Source: CAD feature listing. Evaluate the final solid. Frame: model axes, mm. A direction names the side the tool comes from. Round coordinates to 2 decimals unless told otherwise and drop trailing zeros. Write each loop counter-clockwise with the first axis right and the second up, starting at its lowest first coordinate (ties: lowest second). Pieces come first, ordered by that corner, then holes. Notation, with made-up numbers: M 16,29 L 44,29 A28 ccw 44,65 Z; hole C -1.75,12 d7. An arc over 180 degrees is marked long. Use a Markdown table: item, result.
```python
from build123d import *

# Parameters (mm, degrees)
BOSS_EXTRUDE1_START = -2
SKETCH1_R           = 2.5
BOSS_EXTRUDE1_DEPTH = 5.5
BOSS_EXTRUDE2_REACH = 96.094
SKETCH2_R           = 5.5
SKETCH2_R_2         = 2.5
FILLET1_R           = 1.5


with BuildPart() as part:
    # Sketch1 → Boss-Extrude1 (new body)
    with BuildSketch(Plane(origin=(0, -76.733621845, 0), x_dir=(1, 0, 0), z_dir=(0, 1, 0)).offset(BOSS_EXTRUDE1_START)):
        with BuildLine():
            Line((52.941217068, 9.5), (69.945503657, 9.5))
            ThreePointArc((69.945503657, 9.5), (72.232982212, 8.946059138), (74.01360963, 7.406976744))
            Line((74.01360963, 7.406976744), (76.346988808, 4.141579527))
            ThreePointArc((76.346988808, 4.141579527), (82.014772389, 0.763045112), (88.341217068, 2.637708614))
            ThreePointArc((88.341217068, 2.637708614), (90.254455743, 4.667684765), (91.658842367, 7.07786808))
            Line((91.658842367, 7.07786808), (90.278524492, 7.07786808))
            ThreePointArc((90.278524492, 7.07786808), (89.953291089, 6.475468544), (89.591215146, 5.89446684))
            Line((89.591215146, 5.89446684), (88.341217068, 5.89446684))
            Line((88.341217068, 5.89446684), (88.341217068, 12))
            Line((88.341217068, 12), (88.341217068, 13.810660172))
            ThreePointArc((88.341217068, 13.810660172), (86.557690725, 18.116473657), (82.25187724, 19.9))
            Line((82.25187724, 19.9), (80.441217068, 19.9))
            ThreePointArc((80.441217068, 19.9), (76.827000951, 19.024773438), (74.01360963, 16.593023256))
            ThreePointArc((74.01360963, 16.593023256), (72.232982212, 15.053940862), (69.945503657, 14.5))
            Line((69.945503657, 14.5), (52.941217068, 14.5))
            ThreePointArc((52.941217068, 14.5), (50.441217068, 12), (52.941217068, 9.5))
        make_face()
        with Locations(Location((80.441217068, 12, 0), (0, 0, 270))):
            Circle(SKETCH1_R, mode=Mode.SUBTRACT)
    extrude(amount=-BOSS_EXTRUDE1_DEPTH)

    # Sketch2 → Boss-Extrude2 (add, up to next)
    with BuildSketch(Plane(origin=(0, -76.733621845, 0), x_dir=(-1, 0, 0), z_dir=(0, -1, 0)), mode=Mode.PRIVATE) as boss_extrude2_sk1:
        with Locations(Location((-80.441217068, 12, 0), (0, 0, 270))):
            Circle(SKETCH2_R)
        with Locations(Location((-80.441217068, 12, 0), (0, 0, 270))):
            Circle(SKETCH2_R_2, mode=Mode.SUBTRACT)
    boss_extrude2_tool1 = extrude(boss_extrude2_sk1.sketch, amount=BOSS_EXTRUDE2_REACH, mode=Mode.PRIVATE) - part.part
    add(boss_extrude2_tool1.solids().sort_by_distance((80.441217, -76.733622, -17.344437))[0])

    # Fillet1
    fillet1_edges = [part.edges().sort_by_distance(p)[0] for p in [
        (80.441217068, -78.733621845, -17.5),
    ]]
    fillet(fillet1_edges, radius=FILLET1_R)


solid = part.part
```
Q1. Line query: L1, parallel to X at y = -81.25, z = -12; L2, parallel to Y at x = 83, z = -1.75; L3, parallel to Z at x = 80.5, y = -80.5. Output: solid intervals per line, ascending.
Results are:
| item | result |
|---|---|
| L1 | 50.44 to 77.94, 82.94 to 88.34 |
| L2 | -84.23 to -78.73 |
| L3 | -19.9 to -14.5, -9.5 to -1.1 |
Q2. Section D-D on y = -78. Return loops of the section in (x, z).
Results are:
| item | result |
|---|---|
| outline | C 80.44,-12 d11.42; hole C 80.44,-12 d5 |
Q3. Mould query, pull axis X, two halves, no side actions, for faces 1 (the cylindrical face through (81.921, -81.445, -0.775)), 2 (the flat face through (91, -81, -7.078)), 3 (the flat face through (89, -81, -5.894)). Classes: +X half, -X half, draft (parallel to the pull), parting line (faces both ways), or undercut.
Results are:
| item | result |
|---|---|
| face 1 | parting line |
| face 2 | draft |
| face 3 | undercut |
Q4. Reachability of faces 4 (the flat face through (62, -81, -14.5)), 5 (the cylindrical face through (89.958, -81.445, -6.484)), 6 (the cylindrical face through (86.605, -81.445, -18.069)), 7 (the flat face through (61, -81, -9.5)), 8 (the flat face through (81.6, -76.734, -9.6)) from +Z, -Z, +X, -X, +Y, -Y: full face, straight path, thin tool, end or side. Return the list, or none.
Results are:
| item | result |
|---|---|
| face 4 | -Z, -X, +Y, -Y |
| face 5 | -Z, +Y, -Y |
| face 6 | -Z, +X, +Y, -Y |
| face 7 | +Z, -X, +Y, -Y |
| face 8 | +Z, -Z, +X, -X, +Y |
Q5. Section B-B on y = -81.75. Return loops of the section in (x, z), plus the area to 3 significant figures.
Results are:
| item | result |
|---|---|
| outline | M 52.94,-14.5 L 69.95,-14.5 A5 cw 74.01,-16.59 A7.9 ccw 80.44,-19.9 L 82.25,-19.9 A6.09 ccw 88.34,-13.81 L 88.34,-5.89 L 89.59,-5.89 A11 cw 90.28,-7.08 L 91.66,-7.08 A12.25 ccw 88.34,-2.64 A8.22 ccw 76.35,-4.14 L 74.01,-7.41 A5 cw 69.95,-9.5 L 52.94,-9.5 A2.5 ccw Z; hole C 80.44,-12 d5 |
| area | 346 mm^2 |
Q6. Section A-A on z = -12. Return loops of the section in (x, y), plus the area to 3 significant figures.
Results are:
| item | result |
|---|---|
| outline | M 50.44,-84.23 L 77.94,-84.23 L 77.94,-76.73 L 74.94,-76.73 L 74.94,-77.23 A1.5 cw 73.44,-78.73 L 50.44,-78.73 Z; M 82.94,-84.23 L 88.34,-84.23 L 88.34,-78.73 L 87.44,-78.73 A1.5 cw 85.94,-77.23 L 85.94,-76.73 L 82.94,-76.73 Z |
| area | 194 mm^2 |
Q7. First-contact query: pin 1 Ø1.6 at (x, y) = (62.5, -82) entering from +Z; pin 2 Ø6 at (x, z) = (63, -5.5) entering from -Y; pin 3 Ø2 at (y, z) = (-80, -12) entering from +X; pin 4 Ø9.5 at (x, z) = (80, -5.5) entering from +Y. Flat tips, straight axial feed; report the tip coordinate or a pass-through.
Results are:
| item | result |
|---|---|
| pin 1 | z = -9.5 |
| pin 2 | through |
| pin 3 | x = 88.34 |
| pin 4 | y = -76.73 |
Q8. Section C-C on x = 57.5. Return loops of the section in (y, z).
Results are:
| item | result |
|---|---|
| outline | M -84.23,-14.5 L -78.73,-14.5 L -78.73,-9.5 L -84.23,-9.5 Z |
